```python
from build123d import *

# Parameters (mm, degrees)
SKETCH1_W           = 150
SKETCH1_H           = 150
BOSS_EXTRUDE1_DEPTH = 10
SKETCH2_W           = 40
SKETCH2_H           = 5
SKETCH2_H_2         = 10
BOSS_EXTRUDE2_DEPTH = 10
SKETCH3_W           = 40
SKETCH3_H           = 5
CUT_EXTRUDE1_DEPTH  = 10
SKETCH4_W           = 10
SKETCH4_H           = 150
BOSS_EXTRUDE3_DEPTH = 30


with BuildPart() as part:
    # Sketch1 → Boss-Extrude1 (new body)
    with BuildSketch(Plane.XY):
        with Locations((-31.208053691, -10.570469799)):
            Rectangle(SKETCH1_W, SKETCH1_H)
    extrude(amount=BOSS_EXTRUDE1_DEPTH)

    # Sketch2 → Boss-Extrude2 (add)
    with BuildSketch(Plane.XY.offset(10)):
        Polygon((-96.208053691, 64.429530201), (-106.208053691, 64.429530201), (-106.208053691, -85.570469799), (-96.208053691, -85.570469799), (-96.208053691, -75.570469799), (-96.208053691, -35.570469799), (-96.208053691, -30.570469799), (-96.208053691, 9.429530201), (-96.208053691, 14.429530201), (-96.208053691, 54.429530201), align=None)
        with Locations((-76.208053691, 11.929530201)):
            Rectangle(SKETCH2_W, SKETCH2_H)
        Polygon((-51.208053691, 64.429530201), (-56.208053691, 64.429530201), (-56.208053691, 54.429530201), (-56.208053691, 14.429530201), (-56.208053691, 9.429530201), (-56.208053691, -30.570469799), (-56.208053691, -35.570469799), (-56.208053691, -75.570469799), (-56.208053691, -85.570469799), (-51.208053691, -85.570469799), (-51.208053691, -75.570469799), (-51.208053691, -35.570469799), (-51.208053691, -30.570469799), (-51.208053691, 9.429530201), (-51.208053691, 14.429530201), (-51.208053691, 54.429530201), align=None)
        with Locations((-76.208053691, 59.429530201)):
            Rectangle(SKETCH2_W, SKETCH2_H_2)
        with Locations((-31.208053691, 59.429530201)):
            Rectangle(SKETCH2_W, SKETCH2_H_2)
        Polygon((-6.208053691, 64.429530201), (-11.208053691, 64.429530201), (-11.208053691, 54.429530201), (-11.208053691, 14.429530201), (-11.208053691, 9.429530201), (-11.208053691, -30.570469799), (-11.208053691, -35.570469799), (-11.208053691, -75.570469799), (-11.208053691, -85.570469799), (-6.208053691, -85.570469799), (-6.208053691, -75.570469799), (-6.208053691, -35.570469799), (-6.208053691, -30.570469799), (-6.208053691, 9.429530201), (-6.208053691, 14.429530201), (-6.208053691, 54.429530201), align=None)
        with Locations((13.791946309, 59.429530201)):
            Rectangle(SKETCH2_W, SKETCH2_H_2)
        Polygon((43.791946309, 64.429530201), (33.791946309, 64.429530201), (33.791946309, 54.429530201), (33.791946309, 14.429530201), (33.791946309, 9.429530201), (33.791946309, -30.570469799), (33.791946309, -35.570469799), (33.791946309, -75.570469799), (33.791946309, -85.570469799), (43.791946309, -85.570469799), align=None)
        with Locations((-76.208053691, -80.570469799)):
            Rectangle(SKETCH2_W, SKETCH2_H_2)
        with Locations((13.791946309, -80.570469799)):
            Rectangle(SKETCH2_W, SKETCH2_H_2)
        with Locations((-31.208053691, -80.570469799)):
            Rectangle(SKETCH2_W, SKETCH2_H_2)
        with Locations((-31.208053691, 11.929530201)):
            Rectangle(SKETCH2_W, SKETCH2_H)
        with Locations((13.791946309, 11.929530201)):
            Rectangle(SKETCH2_W, SKETCH2_H)
        with Locations((13.791946309, -33.070469799)):
            Rectangle(SKETCH2_W, SKETCH2_H)
        with Locations((-76.208053691, -33.070469799)):
            Rectangle(SKETCH2_W, SKETCH2_H)
        with Locations((-31.208053691, -33.070469799)):
            Rectangle(SKETCH2_W, SKETCH2_H)
    extrude(amount=BOSS_EXTRUDE2_DEPTH)

    # Sketch3 → Cut-Extrude1 (cut)
    with BuildSketch(Plane.XY.offset(10)):
        with Locations((-76.208053691, 51.929530201)):
            Rectangle(SKETCH3_W, SKETCH3_H)
        with Locations((-31.208053691, 51.929530201)):
            Rectangle(SKETCH3_W, SKETCH3_H)
        with Locations((13.791946309, 51.929530201)):
            Rectangle(SKETCH3_W, SKETCH3_H)
        with Locations((-76.208053691, 6.929530201)):
            Rectangle(SKETCH3_W, SKETCH3_H)
        with Locations((-31.208053691, 6.929530201)):
            Rectangle(SKETCH3_W, SKETCH3_H)
        with Locations((13.791946309, 6.929530201)):
            Rectangle(SKETCH3_W, SKETCH3_H)
        with Locations((-76.208053691, -38.070469799)):
            Rectangle(SKETCH3_W, SKETCH3_H)
        with Locations((-31.208053691, -38.070469799)):
            Rectangle(SKETCH3_W, SKETCH3_H)
        with Locations((13.791946309, -38.070469799)):
            Rectangle(SKETCH3_W, SKETCH3_H)
    extrude(amount=-CUT_EXTRUDE1_DEPTH, mode=Mode.SUBTRACT)

    # Sketch4 → Boss-Extrude3 (add)
    with BuildSketch(Plane(origin=(0, 0, 0), x_dir=(-1, 0, 0), z_dir=(0, 0, -1))):
        with Locations((-38.791946309, -10.570469799)):
            Rectangle(SKETCH4_W, SKETCH4_H)
        with Locations((101.208053691, -10.570469799)):
            Rectangle(SKETCH4_W, SKETCH4_H)
    extrude(amount=BOSS_EXTRUDE3_DEPTH)


solid = part.part
```
Geometry check sheet. Reference: the model listing, model coordinates, mm. A direction names the side the tool comes from. Round coordinates to 2 decimals unless told otherwise and drop trailing zeros. Write each loop counter-clockwise with the first axis right and the second up, starting at its lowest first coordinate (ties: lowest second). Pieces come first, ordered by that corner, then holes. Notation, with made-up numbers: (6, 23) -> (56, 23) arc R21 ccw to (56, 55) -> close; hole circle Ø9 at (36, -19.75). An arc over 180 degrees is marked (long way). Put each result on its own line as item: value.
1) Cross-section at A-A, the plane z = -21. Enter the section's corners in (x, y), plus the area to 3 significant figures.
Recorded:
outline: (-106.21, -85.57) -> (-96.21, -85.57) -> (-96.21, 64.43) -> (-106.21, 64.43) -> close; (33.79, -85.57) -> (43.79, -85.57) -> (43.79, 64.43) -> (33.79, 64.43) -> close
area: 3,000 mm2
2) Release check for a two-part mould opening along Y. For faces 3 (the face through (-76, 14.43, 15)), 4 (the face through (-31, 14.43, 15)) record: pulls with the +Y half, pulls with the -Y half, needs draft (parallel to the pull), parting line crosses it, or undercut.
Recorded:
face 3: undercut
face 4: undercut
3) Depth check by flat-ended pin: P1, Ø1.5, axis at x = 17.5, y = 26.5, coming from the +Z side; P2, Ø12, axis at x = -50, y = -18.5, coming from the -Z side. Enter the tip coordinate at first touch or a pass-through.
Recorded:
P1: stops at z = 10
P2: stops at z = 0
4) Access from +Z, -Z, +X, -X, +Y, -Y to the whole of each face (thin tool, end or side, straight path). Record for faces 1 (the face through (-31, 4.43, 5)), 2 (the face through (-6.208, 34, 14)).
Recorded:
face 1: +Z, -Z
face 2: +Z
5) Thickness scan on probe 1 along Y at (x, z) = (-23, 3.5); probe 2 along X at (y, z) = (19, 16); probe 3 along Y at (x, z) = (-60, 13). Record the ranges inside material, lowest first. Write a range as from..to.
Recorded:
probe 1: y = -85.57..-40.57, -35.57..4.43, 9.43..49.43, 54.43..64.43
probe 2: x = -106.21..-96.21, -56.21..-51.21, -11.21..-6.21, 33.79..43.79
probe 3: y = -85.57..-75.57, -35.57..-30.57, 9.43..14.43, 54.43..64.43
6) Cross-section at D-D, the plane z = 8. Give the number of separate pieces and of enclosed holes in the cut face, plus the area to 3 significant figures.
Recorded:
separate pieces: 1
enclosed holes: 9
area: 20,700 mm2
7) Cross-section at C-C, the plane y = -33. Enter the section's corners in (x, z).
Recorded:
outline: (-106.21, -30) -> (-96.21, -30) -> (-96.21, 0) -> (33.79, 0) -> (33.79, -30) -> (43.79, -30) -> (43.79, 20) -> (-106.21, 20) -> close
8) Cross-section at B-B, the plane x = -86.5. Enter the section's corners in (y, z).
Recorded:
outline: (-85.57, 0) -> (-40.57, 0) -> (-40.57, 10) -> (-75.57, 10) -> (-75.57, 20) -> (-85.57, 20) -> close; (-35.57, 0) -> (4.43, 0) -> (4.43, 10) -> (-30.57, 10) -> (-30.57, 20) -> (-35.57, 20) -> close; (9.43, 0) -> (49.43, 0) -> (49.43, 10) -> (14.43, 10) -> (14.43, 20) -> (9.43, 20) -> close; (54.43, 0) -> (64.43, 0) -> (64.43, 20) -> (54.43, 20) -> close
